Build history of the part. All positions in model axes, mm. A direction names the side the tool comes from. Give positions to 0.01 mm unless a question says otherwise; leave off trailing zeros. Order: outer loops, then holes, each group sorted by start corner. A loop starts at its lowest first (then second) coordinate and runs counter-clockwise, first axis right, second up. Notation, with made-up numbers: (20, 20.25) - (43, 20.25) arc R34 ccw to (43, 53.25) - close; hole circle Ø3 at (54.25, 75). An arc over 180 degrees is marked (long way). Answer in a Markdown table with one row per item.
```python
from build123d import *

# Parameters (mm, degrees)
SKETCH1_R           = 5.75
BOSS_EXTRUDE1_DEPTH = 15
CUT_EXTRUDE3_DEPTH  = 8
SKETCH7_R           = 1
CUT_EXTRUDE4_DEPTH  = 6.5


with BuildPart() as part:
    # Sketch1 → Boss-Extrude1 (new body)
    with BuildSketch(Plane(origin=(0, 0, 0), x_dir=(1, 0, 0), z_dir=(0, 1, 0))):
        with Locations(Location((0, 0, 0), (0, 0, 270))):
            Circle(SKETCH1_R)
    extrude(amount=BOSS_EXTRUDE1_DEPTH)

    # Sketch6 → Cut-Extrude3 (cut)
    with BuildSketch(Plane(origin=(0, 15, 0), x_dir=(1, 0, 0), z_dir=(0, 1, 0))):
        with BuildLine():
            Line((0.41, 2.964671599), (0.41, -2.964671599))
            ThreePointArc((0.41, -2.964671599), (3.374671599, 0), (0.41, 2.964671599))
        make_face()
        with BuildLine():
            Line((-0.416408681, 2.965564682), (-0.416408681, -2.965564682))
            ThreePointArc((-0.416408681, -2.965564682), (-3.381973363, 0), (-0.416408681, 2.965564682))
        make_face()
    extrude(amount=-CUT_EXTRUDE3_DEPTH, mode=Mode.SUBTRACT)

    # Sketch7 → Cut-Extrude4 (cut)
    with BuildSketch(Plane(origin=(0, 0, 0), x_dir=(1, 0, 0), z_dir=(0, 1, 0))):
        with Locations(Location((0, 0, 0), (0, 0, 90))):
            Circle(SKETCH7_R)
    extrude(amount=CUT_EXTRUDE4_DEPTH, mode=Mode.SUBTRACT)


solid = part.part
```
1. Which spindle directions (+Z, -Z, +X, -X, +Y, -Y) get a long thin tool onto all of the face, cutting with end or side? Do faces 4 (the face through (3.374, 11.056, 0.065)), 5 (the face through (0, 6.5, 0)), 6 (the face through (0.1, 0, 1.2)). Say none if no direction does.
Check result:
| item | result |
|---|---|
| face 4 | +Y |
| face 5 | -Y |
| face 6 | +Z, -Z, +X, -X, -Y |
2. Cut at A-A on x = 0. Write the cut outline in (y, z).
Check result:
| item | result |
|---|---|
| outline | (0, -5.75) - (15, -5.75) - (15, 5.75) - (0, 5.75) - (0, 1) - (6.5, 1) - (6.5, -1) - (0, -1) - close |
3. Probe line 1 (X direction, y = 8, z = -1); line 2 (X direction, y = 2.25, z = 0); line 3 (Y direction, x = 2.5, z = 0.5). List the from-to ranges inside material, lowest first.
Check result:
| item | result |
|---|---|
| line 1 | x = -5.66 to -3.21, -0.42 to 0.41, 3.2 to 5.66 |
| line 2 | x = -5.75 to -1, 1 to 5.75 |
| line 3 | y = 0 to 7 |
4. Cut at D-D on y = 9. Write the cut outline in (x, z).
Check result:
| item | result |
|---|---|
| outline | circle Ø11.5 at (0, 0); hole (-0.42, -2.97) - (-0.42, 2.97) arc R2.97 ccw to start; hole (0.41, -2.96) arc R2.96 ccw to (0.41, 2.96) - close |
5. Drop flat-ended pins along their axis: P1, Ø3.5, axis at x = -2.5, z = 0.5, coming from the +Y side; P2, Ø1.5, axis at y = 1.5, z = 2, coming from the -X side; P3, Ø2, axis at x = -2, z = -1, coming from the +Y side; P4, Ø2, axis at y = 2.5, z = -2, coming from the -X side. Give the stop position or say it passes through.
Check result:
| item | result |
|---|---|
| P1 | stops at y = 15 |
| P2 | stops at x = -5.61 |
| P3 | stops at y = 7 |
| P4 | stops at x = -5.66 |
6. Two-plate mould, pull along Z, no slides. Class faces 1 (the face through (4.85, 7.4, 3.09)), 2 (the face through (1, 3, 0)), 3 (the face through (0, 15, 0)): +Z half, -Z half, draft (parallel to the pull), parting line (faces both ways), or undercut.
Check result:
| item | result |
|---|---|
| face 1 | parting line |
| face 2 | undercut |
| face 3 | draft |
7. Cut at B-B on z = 0. Write the cut outline in (x, y).
Check result:
| item | result |
|---|---|
| outline | (-5.75, 0) - (-1, 0) - (-1, 6.5) - (1, 6.5) - (1, 0) - (5.75, 0) - (5.75, 15) - (3.37, 15) - (3.37, 7) - (0.41, 7) - (0.41, 15) - (-0.42, 15) - (-0.42, 7) - (-3.38, 7) - (-3.38, 15) - (-5.75, 15) - close |
8. Cut at C-C on y = 5. Write the cut outline in (x, z), and give its area (3 significant figures).
Check result:
| item | result |
|---|---|
| outline | circle Ø11.5 at (0, 0); hole circle Ø2 at (0, 0) |
| area | 101 mm² |
